Work out the finished part from the listing and answer in its coordinate system (mm). A direction names the side the tool comes from. Round coordinates to 2 decimals unless told otherwise and drop trailing zeros. Order: outer loops, then holes, each group sorted by start corner. A loop starts at its lowest first (then second) coordinate and runs counter-clockwise, first axis right, second up. Notation, with made-up numbers: (-31.75, 77.5) - (-21.75, 77.5) arc R29 ccw to (-21.75, 115.5) - close; hole circle Ø3 at (15, -12.75). An arc over 180 degrees is marked (long way). Put each result on its own line as item: value.
```python
from build123d import *

# Parameters (mm, degrees)
BOSS_EXTRUDE1_DEPTH = 4
CUT_EXTRUDE1_DEPTH  = 10


with BuildPart() as part:
    # Sketch1 → Boss-Extrude1 (new body)
    with BuildSketch(Plane(origin=(0, 0, 0), x_dir=(1, 0, 0), z_dir=(0, 1, 0))):
        Polygon((-148, 18.23), (-148, 6), (-152, 6), (-152, 2), (-148, 2), (-148, -10), (-152, -10), (-152, -14), (-148, -14), (-148, -17.38), (-52, -17.38), (-52, -3.77), (-48, -3.77), (-48, 0.23), (-52, 0.23), (-52, 12.23), (-48, 12.23), (-48, 16.23), (-52, 16.23), (-52, 18.23), align=None)
    extrude(amount=-BOSS_EXTRUDE1_DEPTH)

    # Sketch2 → Cut-Extrude1 (cut)
    with BuildSketch(Plane(origin=(0, 0, 0), x_dir=(1, 0, 0), z_dir=(0, 1, 0))):
        with BuildLine():
            ThreePointArc((-144, 7.862318396), (-143.26536282, 9.411142768), (-141.601143065, 9.822143171))
            Line((-141.601143065, 9.822143171), (-122.254722174, 5.884824774))
            ThreePointArc((-122.254722174, 5.884824774), (-120.663648262, 3.724562414), (-122.653579109, 1.925))
            Line((-122.653579109, 1.925), (-142, 1.925))
            ThreePointArc((-142, 1.925), (-143.414213562, 2.510786438), (-144, 3.925))
            Line((-144, 3.925), (-144, 7.862318396))
        make_face()
        with BuildLine():
            Line((-123.346420891, 14.23), (-104, 14.23))
            ThreePointArc((-104, 14.23), (-102.585786438, 13.644213562), (-102, 12.23))
            Line((-102, 12.23), (-102, 8.292681604))
            ThreePointArc((-102, 8.292681604), (-102.73463718, 6.743857232), (-104.398856935, 6.332856829))
            Line((-104.398856935, 6.332856829), (-123.745277826, 10.270175226))
            ThreePointArc((-123.745277826, 10.270175226), (-125.336351738, 12.430437586), (-123.346420891, 14.23))
        make_face()
        with BuildLine():
            Line((-98, 12.23), (-98, 8.292681604))
            ThreePointArc((-98, 8.292681604), (-97.26536282, 6.743857232), (-95.601143065, 6.332856829))
            Line((-95.601143065, 6.332856829), (-76.254722174, 10.270175226))
            ThreePointArc((-76.254722174, 10.270175226), (-74.663648262, 12.430437586), (-76.653579109, 14.23))
            Line((-76.653579109, 14.23), (-96, 14.23))
            ThreePointArc((-96, 14.23), (-97.414213562, 13.644213562), (-98, 12.23))
        make_face()
        with BuildLine():
            ThreePointArc((-56, 3.925), (-56.585786438, 2.510786438), (-58, 1.925))
            Line((-58, 1.925), (-77.346420891, 1.925))
            ThreePointArc((-77.346420891, 1.925), (-79.336351738, 3.724562414), (-77.745277826, 5.884824774))
            Line((-77.745277826, 5.884824774), (-58.398856935, 9.822143171))
            ThreePointArc((-58.398856935, 9.822143171), (-56.73463718, 9.411142768), (-56, 7.862318396))
            Line((-56, 7.862318396), (-56, 3.925))
        make_face()
        with BuildLine():
            ThreePointArc((-56, -7.012318396), (-56.73463718, -8.561142768), (-58.398856935, -8.972143171))
            Line((-58.398856935, -8.972143171), (-77.745277826, -5.034824774))
            ThreePointArc((-77.745277826, -5.034824774), (-79.336351738, -2.874562414), (-77.346420891, -1.075))
            Line((-77.346420891, -1.075), (-58, -1.075))
            ThreePointArc((-58, -1.075), (-56.585786438, -1.660786438), (-56, -3.075))
            Line((-56, -3.075), (-56, -7.012318396))
        make_face()
        with BuildLine():
            Line((-76.653579109, -13.38), (-96, -13.38))
            ThreePointArc((-96, -13.38), (-97.414213562, -12.794213562), (-98, -11.38))
            Line((-98, -11.38), (-98, -7.442681604))
            ThreePointArc((-98, -7.442681604), (-97.26536282, -5.893857232), (-95.601143065, -5.482856829))
            Line((-95.601143065, -5.482856829), (-76.254722174, -9.420175226))
            ThreePointArc((-76.254722174, -9.420175226), (-74.663648262, -11.580437586), (-76.653579109, -13.38))
        make_face()
        with BuildLine():
            ThreePointArc((-144, -3.075), (-143.414213562, -1.660786438), (-142, -1.075))
            Line((-142, -1.075), (-122.653579109, -1.075))
            ThreePointArc((-122.653579109, -1.075), (-120.663648262, -2.874562414), (-122.254722174, -5.034824774))
            Line((-122.254722174, -5.034824774), (-141.601143065, -8.972143171))
            ThreePointArc((-141.601143065, -8.972143171), (-143.26536282, -8.561142768), (-144, -7.012318396))
            Line((-144, -7.012318396), (-144, -3.075))
        make_face()
        with BuildLine():
            Line((-104.398856935, -5.482856829), (-123.745277826, -9.420175226))
            ThreePointArc((-123.745277826, -9.420175226), (-125.336351738, -11.580437586), (-123.346420891, -13.38))
            Line((-123.346420891, -13.38), (-104, -13.38))
            ThreePointArc((-104, -13.38), (-102.585786438, -12.794213562), (-102, -11.38))
            Line((-102, -11.38), (-102, -7.442681604))
            ThreePointArc((-102, -7.442681604), (-102.73463718, -5.893857232), (-104.398856935, -5.482856829))
        make_face()
    extrude(amount=-CUT_EXTRUDE1_DEPTH, mode=Mode.SUBTRACT)


solid = part.part
```
1) A cutting plane is placed at A-A on x = -116.5. Write down the section's boundary in (y, z).
Findings below:
outline: (-4, -18.23) - (0, -18.23) - (0, -14.23) - (-4, -14.23) - close; (-4, -8.8) - (0, -8.8) - (0, 7.95) - (-4, 7.95) - close; (-4, 13.38) - (0, 13.38) - (0, 17.38) - (-4, 17.38) - close
2) A cutting plane is placed at C-C on y = -1.7. Give the number of separate pieces and of enclosed holes in the cut face, then the cut area to 3 significant figures.
Findings below:
separate pieces: 1
enclosed holes: 8
area: 2,390 mm2
3) Given pin 1 Ø1.2 at (x, y) = (-149.5, -1.5) entering from +Z; pin 2 Ø2 at (x, y) = (-150, -1.5) entering from -Z; pin 3 Ø2 at (x, y) = (-50, -2) entering from -Z, each flat-ended and moving along its own axis, determine where each tip first touches the part or whether it passes through.
Findings below:
pin 1: stops at z = 14
pin 2: stops at z = -6
pin 3: stops at z = -16.23
4) For faces 5 (the flat face through (-50, -2, -0.23)), 6 (the cylindrical face through (-125.34, -1.97, -12.39)), 7 (the flat face through (-150, -2, 14)), 8 (the flat face through (-150, -2, -2)), determine the directions among +Z, -Z, +X, -X, +Y, -Y from which every point of the face is accessible in a straight line to the end or side of a thin tool.
Findings below:
face 5: +X, +Y, -Y
face 6: +Y, -Y
face 7: +Z, -X, +Y, -Y
face 8: -X, +Y, -Y
5) A cutting plane is placed at B-B on z = -3. Write down the section's boundary in (x, y).
Findings below:
outline: (-152, -4) - (-143.77, -4) - (-143.77, 0) - (-152, 0) - close; (-120.88, -4) - (-79.12, -4) - (-79.12, 0) - (-120.88, 0) - close; (-56.23, -4) - (-52, -4) - (-52, 0) - (-56.23, 0) - close
6) For a pull along Z with two mould halves and no side action, classify faces 1 (the flat face through (-101, 0, -1)), 2 (the cylindrical face through (-143.28, -1.97, -9.4)), 3 (the cylindrical face through (-97.284, -1.972, 5.91)), 4 (the flat face through (-101, -2, 17.38)) as pulls with the +Z half, pulls with the -Z half, needs draft (parallel to the pull), parting line crosses it, or undercut.
Findings below:
face 1: needs draft
face 2: undercut
face 3: undercut
face 4: pulls with the +Z half
7) Straight lines are drawn through the part: L1, parallel to Z at x = -95.5, y = -2.8; L2, parallel to X at y = -3.25, z = 3; L3, parallel to X at y = -2, z = 11.5. For each, find the intervals that lie inside material, in ascending order. Write a range as from..to.
Findings below:
L1: z = -18.23..-14.23, -6.35..5.5, 13.38..17.38
L2: x = -148..-144, -120.65..-79.35, -56..-48
L3: x = -152..-125.34, -102..-98, -74.66..-52
